CAD build for the part. Positions are in the model's coordinates, mm. Give positions to 0.01 mm unless a question says otherwise; leave off trailing zeros. Order: outer loops, then holes, each group sorted by start corner. A loop starts at its lowest first (then second) coordinate and runs counter-clockwise, first axis right, second up. Notation, with made-up numbers: (-28.75, 64.25) -> (23.25, 64.25) arc R16 ccw to (23.25, 91.25) -> close; hole circle Ø1 at (3.25, 21.5). An arc over 180 degrees is marked (long way). Answer as CSV lines item,"result".
```python
from build123d import *

# Parameters (mm, degrees)
F0_R     = 7.664283
F1_DEPTH = 25.4


with BuildPart() as f1:
    # F0 (on Front) → F1 (new body)
    with BuildSketch(Plane.XZ):
        Polygon((41.265003, 42.209998), (-54.18, 42.209998), (-48.824999, -24.255), (41.265003, -24.255), align=None)
        with BuildLine():
            ThreePointArc((-21.381332, 14.608613), (-13.495042, 36.008892), (4.780889, 22.364998))
            ThreePointArc((4.780889, 22.364998), (1.11502, 12.830925), (-7.993936, 8.208795))
            ThreePointArc((-7.993936, 8.208795), (-18.911873, 2.57227), (-21.381332, 14.608613))
        make_face(mode=Mode.SUBTRACT)
        with Locations((-34.019999, 29.295001)):
            Circle(F0_R, mode=Mode.SUBTRACT)
    extrude(amount=F1_DEPTH)


solid = f1.part
```
1) Band-saw the part on A-A, the plane x = -11.5. Write the cut outline in (y, z) (3 decimals).
Data:
outline,"(-25.4, -24.255) -> (0, -24.255) -> (0, 2.992) -> (-25.4, 2.992) -> close; (-25.4, 36.447) -> (0, 36.447) -> (0, 42.21) -> (-25.4, 42.21) -> close"
2) Pull direction X, two halves, no side cores. Call faces 1 (the flat face through (-7, 0, 2)), 2 (the cylindrical face through (-18.73, -12.52, 2.49)), 3 (the flat face through (-51.54, -12.52, 9.44)): pulls with the +X half, pulls with the -X half, needs draft (parallel to the pull), parting line crosses it, or undercut.
Data:
face 1,"needs draft"
face 2,"undercut"
face 3,"pulls with the -X half"
3) Band-saw the part on D-D, the plane z = 4. Write the cut outline in (x, y) (3 decimals), then the cut area to 3 significant figures.
Data:
outline,"(-51.101, -25.4) -> (-20.961, -25.4) -> (-20.961, 0) -> (-51.101, 0) -> close; (-10.215, -25.4) -> (41.265, -25.4) -> (41.265, 0) -> (-10.215, 0) -> close"
area,"2,070 mm2"
4) Pin check, flat tips, straight feed: P1, Ø1.5, axis at y = -16, z = 11.5, coming from the -X side; P2, Ø5, axis at y = -16, z = 29, coming from the -X side; P3, Ø8, axis at y = -8, z = 14.5, coming from the -X side. Stop position of each tip, or through.
Data:
P1,"stops at x = -51.77"
P2,"stops at x = -53.32"
P3,"stops at x = -52.27"
5) Band-saw the part on B-B, the plane y = -14.25. Write the cut outline in (x, z) (3 decimals), then the cut area to 3 significant figures.
Data:
outline,"(-54.18, 42.21) -> (-48.825, -24.255) -> (41.265, -24.255) -> (41.265, 42.21) -> close; hole circle Ø15.329 at (-34.02, 29.295); hole (-21.381, 14.609) arc R7.707 ccw (long way) to (-7.994, 8.209) arc R14.231 ccw (long way) to start"
area,"5,240 mm2"
6) Band-saw the part on C-C, the plane z = 33. Write the cut outline in (x, y) (3 decimals), then the cut area to 3 significant figures.
Data:
outline,"(-53.438, -25.4) -> (-40.729, -25.4) -> (-40.729, 0) -> (-53.438, 0) -> close; (-27.311, -25.4) -> (-18.906, -25.4) -> (-18.906, 0) -> (-27.311, 0) -> close; (0.006, -25.4) -> (41.265, -25.4) -> (41.265, 0) -> (0.006, 0) -> close"
area,"1,580 mm2"
7) Wall check: line 1 along X through (y, z) = (-17.75, 35) (3 decimals); line 2 along Z through (x, y) = (-32, -5.5) (3 decimals); line 3 along Z through (x, y) = (-13.5, -1.5) (3 decimals). Give the ranges that are in metal, low to high. Write a range as [from, to].
Data:
line 1,"x = [-53.599, -39.138], [-28.902, -15.998], [-2.902, 41.265]"
line 2,"z = [-24.255, 21.902], [36.688, 42.21]"
line 3,"z = [-24.255, 2.107], [36.007, 42.21]"
